Check sheet for the modelled part. Datum: model origin and axes. Units: mm. A direction names the side the tool comes from. Round coordinates to 2 decimals unless told otherwise and drop trailing zeros. Order: outer loops, then holes, each group sorted by start corner. A loop starts at its lowest first (then second) coordinate and runs counter-clockwise, first axis right, second up.
```python
from build123d import *

# Parameters (mm, degrees)
F0_W     = 915
F0_H     = 2200
F1_DEPTH = 600
F2_W     = 755
F2_H     = 220
F2_H_2   = 300
F2_H_3   = 211.888492
F2_H_4   = 180.111508
F3_DEPTH = 600


with BuildPart() as f1:
    # F0 (on Front) → F1 (new body)
    with BuildSketch(Plane.XZ):
        Rectangle(F0_W, F0_H)
    extrude(amount=F1_DEPTH)

    # F2 (on face) → F3 (cut, through all)
    with BuildSketch(Plane.XZ.offset(600)):
        with Locations((0, 910)):
            Rectangle(F2_W, F2_H)
        with Locations((0, 600)):
            Rectangle(F2_W, F2_H_2)
        with Locations((0, 250)):
            Rectangle(F2_W, F2_H_2)
        with Locations((0, -100)):
            Rectangle(F2_W, F2_H_2)
        with Locations((0, -450)):
            Rectangle(F2_W, F2_H_2)
        with Locations((0, -755.944246)):
            Rectangle(F2_W, F2_H_3)
        with Locations((0, -1001.944246)):
            Rectangle(F2_W, F2_H_4)
    extrude(amount=-F3_DEPTH, mode=Mode.SUBTRACT)


solid = f1.part
```
Item 1: Access from +Z, -Z, +X, -X, +Y, -Y to the whole of each face (thin tool, end or side, straight path). Record for faces 4 (the flat face through (-5, -304, -1092)), 5 (the flat face through (-409, 0, -76)).
Answer:
face 4: +Y, -Y
face 5: +Z, -Z, +X, -X, +Y
Item 2: Sectioned sample at B-B (z = -751.5). Record the cut outline in (x, y), and give its area (3 significant figures).
Answer:
outline: (-457.5, -600) - (-377.5, -600) - (-377.5, 0) - (-457.5, 0) - close; (377.5, -600) - (457.5, -600) - (457.5, 0) - (377.5, 0) - close
area: 96,000 mm2
Item 3: Sectioned sample at A-A (x = -132). State how many separate pieces and enclosed holes the cut face has, and give its area (3 significant figures).
Answer:
separate pieces: 8
enclosed holes: 0
area: 233,000 mm2
Item 4: Release check for a two-part mould opening along Z. For faces 1 (the flat face through (-377.5, -304, -452)), 2 (the flat face through (457.5, -296, -15)), 3 (the flat face through (-6, -296, -1100)) record: released by +Z, released by -Z, zero draft, split by the parting line, or undercut.
Answer:
face 1: undercut
face 2: zero draft
face 3: released by -Z
Item 5: Scan line: line 1 along X through (y, z) = (-533.5, -586). Record every from-to range of solid material in increasing order.
Answer:
line 1: x = -457.5 to -377.5, 377.5 to 457.5
